from build123d import *

# Parameters (mm, degrees)
BOSS_EXTRUDE1_DEPTH = 1.524


with BuildPart() as part:
    # Sketch1 → Boss-Extrude1 (new body)
    with BuildSketch(Plane.XY):
        with BuildLine():
            Line((189.777315793, 495.507175139), (191.224820624, 495.924635056))
            Line((191.224820624, 495.924635056), (196.119223328, 478.946810438))
            ThreePointArc((196.119223328, 478.946810438), (196.281524624, 478.657917117), (196.555651913, 478.471757801))
            ThreePointArc((196.555651913, 478.471757801), (199.147753156, 478.005869728), (201.730327533, 478.521960937))
            ThreePointArc((201.730327533, 478.521960937), (202.122931571, 478.905936562), (202.132531096, 479.455011294))
            Line((202.132531096, 479.455011294), (194.696378786, 494.588452914))
            Line((194.696378786, 494.588452914), (196.085953758, 495.269690236))
            Line((196.085953758, 495.269690236), (203.4004902, 480.349637502))
            ThreePointArc((203.4004902, 480.349637502), (203.905544625, 479.909328052), (204.555334637, 480.072806873))
            ThreePointArc((204.555334637, 480.072806873), (206.275233543, 480.984321258), (208.221715491, 480.995218384))
            ThreePointArc((208.221715491, 480.995218384), (214.599649086, 482.633856482), (218.454712821, 487.972550644))
            ThreePointArc((218.454712821, 487.972550644), (219.175843378, 489.780555467), (220.652597524, 491.048667416))
            ThreePointArc((220.652597524, 491.048667416), (221.042127495, 491.593845171), (220.816722181, 492.224832356))
            Line((220.816722181, 492.224832356), (209.599367356, 504.483762477))
            Line((209.599367356, 504.483762477), (210.741099412, 505.528487706))
            Line((210.741099412, 505.528487706), (222.112676203, 493.07840105))
            ThreePointArc((222.112676203, 493.07840105), (222.627317714, 492.886778176), (223.128167093, 493.112000535))
            ThreePointArc((223.128167093, 493.112000535), (224.551927983, 495.327614554), (225.065041618, 497.910782173))
            ThreePointArc((225.065041618, 497.910782173), (224.99187518, 498.233965919), (224.782226996, 498.490575936))
            Line((224.782226996, 498.490575936), (210.765290937, 509.248234144))
            Line((210.765290937, 509.248234144), (211.682631799, 510.443235718))
            Line((211.682631799, 510.443235718), (223.328487329, 501.504872294))
            ThreePointArc((223.328487329, 501.504872294), (226.03151825, 500.838137649), (228.73454917, 501.504872294))
            ThreePointArc((228.73454917, 501.504872294), (226.018822109, 502.512994153), (223.768735069, 504.337436936))
            ThreePointArc((223.768735069, 504.337436936), (214.697892634, 511.126772614), (205.306886221, 517.465878226))
            ThreePointArc((205.306886221, 517.465878226), (198.926193665, 518.755629479), (192.444429164, 518.152782293))
            ThreePointArc((192.444429164, 518.152782293), (191.977714673, 517.727994557), (192.022339489, 517.098490258))
            Line((192.022339489, 517.098490258), (201.361944543, 503.400969482))
            Line((201.361944543, 503.400969482), (200.088434986, 502.532398479))
            Line((200.088434986, 502.532398479), (190.651660212, 516.372267313))
            ThreePointArc((190.651660212, 516.372267313), (190.110139611, 516.517556306), (189.627566711, 516.232114806))
            ThreePointArc((189.627566711, 516.232114806), (186.698797428, 510.418423529), (185.568771317, 504.007515889))
            ThreePointArc((185.568771317, 504.007515889), (188.039633015, 492.949934603), (191.046560533, 482.025940447))
            ThreePointArc((191.046560533, 482.025940447), (191.923055704, 479.264919011), (191.869552453, 476.368607468))
            ThreePointArc((191.869552453, 476.368607468), (193.477546562, 478.641329665), (193.844210588, 481.401124718))
            Line((193.844210588, 481.401124718), (189.777315793, 495.507175139))
        make_face()
    extrude(amount=BOSS_EXTRUDE1_DEPTH)


solid = part.part
Part model, mm, in its own coordinate system. A direction names the side the tool comes from. Coordinates: 2 decimals unless noted, no trailing zeros. Order: outer loops, then holes, each group sorted by start corner. A loop starts at its lowest first (then second) coordinate and runs counter-clockwise, first axis right, second up. Notation, with made-up numbers: (15, 24) - (39, 24) arc R18 cw to (39, 43) - close; hole circle Ø10 at (82.5, 40). An arc over 180 degrees is marked (long way). Use CSV: the item, a comma, the result in double quotes.
Item 1: 3-axis set-ups, long thin cutter, end or side, ignore diameter. For faces 4 (the face through (202, 498, 1.524)), 5 (the face through (191.839, 488.355, 0.751)): which of +Z, -Z, +X, -X, +Y, -Y reach the whole face in a straight line?
Solved:
face 4,"+Z, +X, -X, +Y, -Y"
face 5,"+Z, -Z"
Item 2: Saw through at B-B on y = 513.5. Give the cut face in (x, z), and give its area (3 significant figures).
Solved:
outline,"(187.98, 0) - (192.61, 0) - (192.61, 1.52) - (187.98, 1.52) - close; (194.48, 0) - (211.3, 0) - (211.3, 1.52) - (194.48, 1.52) - close"
area,"32.7 mm²"
Item 3: Probe probe 1 along X at (y, z) = (495, 0.9); probe 2 along X at (y, z) = (508, 0.65); probe 3 along X at (y, z) = (509.5, 1.2). List the from-to ranges inside material, lowest first.
Solved:
probe 1,"x = 187.54 to 189.92, 191.49 to 195.54, 196.22 to 218.28, 220.36 to 224.41"
probe 2,"x = 186.04 to 196.36, 198.23 to 212.39, 214.87 to 218.99"
probe 3,"x = 186.42 to 195.34, 197.2 to 210.96, 212.91 to 216.96"
Item 4: Saw through at A-A on x = 198.5. Give the cut face in (y, z).
Solved:
outline,"(478.03, 0) - (486.85, 0) - (486.85, 1.52) - (478.03, 1.52) - close; (490.35, 0) - (504.86, 0) - (504.86, 1.52) - (490.35, 1.52) - close; (507.6, 0) - (518.77, 0) - (518.77, 1.52) - (507.6, 1.52) - close"
Item 5: Mould opens along Y. For faces 1 (the face through (211.22, 509.84, 0.75)), 2 (the face through (206.249, 480.978, 0.751)), 3 (the face through (202, 498, 0)) say: +Y half, -Y half, draft (parallel to the pull), parting line (faces both ways), or undercut.
Solved:
face 1,"undercut"
face 2,"-Y half"
face 3,"draft"
Item 6: Saw through at C-C on x = 216.5. Give the cut face in (y, z).
Solved:
outline,"(484.34, 0) - (496.94, 0) - (496.94, 1.52) - (484.34, 1.52) - close; (499.22, 0) - (504.85, 0) - (504.85, 1.52) - (499.22, 1.52) - close; (506.75, 0) - (509.83, 0) - (509.83, 1.52) - (506.75, 1.52) - close"
